Can you work these out from the model? Positions are in its coordinate system, mm. A direction names the side the tool comes from. Round coordinates to 2 decimals unless told otherwise and drop trailing zeros. Order: outer loops, then holes, each group sorted by start corner. A loop starts at its lowest first (then second) coordinate and runs counter-clockwise, first axis right, second up. Notation, with made-up numbers: M -25,9.5 L -8,9.5 A15 cw -8,27.5 Z; hole C 41,63.25 d4. An arc over 180 degrees is marked long. Answer as a JSON object with one key per item and string values. Group by question number.
```python
from build123d import *

# Parameters (mm, degrees)
SKIZZE1_R                       = 23.4
SKIZZE1_R_2                     = 1
LINEAR_AUSTRAGEN1_DEPTH         = 2.2
SKIZZE3_R                       = 1.75
SCHNITT_LINEAR_AUSTRAGEN3_DEPTH = 34.165644875
SKETCH1_R                       = 5
CUT_EXTRUDE1_DEPTH              = 3


with BuildPart() as part:
    # Skizze1 → Linear austragen1 (new body)
    with BuildSketch(Plane.XY):
        Circle(SKIZZE1_R)
        with Locations((6.643865379, 20.4477151)):
            Circle(SKIZZE1_R_2, mode=Mode.SUBTRACT)
        with Locations((17.393865379, 12.637382924)):
            Circle(SKIZZE1_R_2, mode=Mode.SUBTRACT)
        with Locations((17.393865379, -12.637382924)):
            Circle(SKIZZE1_R_2, mode=Mode.SUBTRACT)
        with Locations((-6.643865379, 20.4477151)):
            Circle(SKIZZE1_R_2, mode=Mode.SUBTRACT)
        with Locations((6.643865379, -20.4477151)):
            Circle(SKIZZE1_R_2, mode=Mode.SUBTRACT)
        with Locations((-6.643865379, -20.4477151)):
            Circle(SKIZZE1_R_2, mode=Mode.SUBTRACT)
        with Locations((-17.393865379, -12.637382924)):
            Circle(SKIZZE1_R_2, mode=Mode.SUBTRACT)
        with Locations((-17.393865379, 12.637382924)):
            Circle(SKIZZE1_R_2, mode=Mode.SUBTRACT)
        with BuildLine():
            ThreePointArc((14.720859381, 11.20474449), (0, 18.5), (-14.720859381, 11.20474449))
            ThreePointArc((-14.720859381, 11.20474449), (-14.883940446, 9.033399462), (-12.967323579, 8))
            ThreePointArc((-12.967323579, 8), (0, 8.526339105), (12.967323579, 8))
            ThreePointArc((12.967323579, 8), (14.883940446, 9.033399462), (14.720859381, 11.20474449))
        make_face(mode=Mode.SUBTRACT)
        with BuildLine():
            ThreePointArc((-14.720859381, -11.20474449), (0, -18.5), (14.720859381, -11.20474449))
            ThreePointArc((14.720859381, -11.20474449), (14.883940446, -9.033399462), (12.967323579, -8))
            ThreePointArc((12.967323579, -8), (0, -8.526339105), (-12.967323579, -8))
            ThreePointArc((-12.967323579, -8), (-14.883940446, -9.033399462), (-14.720859381, -11.20474449))
        make_face(mode=Mode.SUBTRACT)
    extrude(amount=LINEAR_AUSTRAGEN1_DEPTH)

    # Skizze3 → Schnitt-Linear austragen3 (cut, through all)
    with BuildSketch(Plane.XY.offset(2.2)):
        with Locations((12.5, 0)):
            Circle(SKIZZE3_R)
        with Locations(Location((-12.5, 0, 0), (0, 0, 180))):
            Circle(SKIZZE3_R)
        with BuildLine():
            Line((-7.295576741, 5.75), (7.295576741, 5.75))
            ThreePointArc((7.295576741, 5.75), (9.59371007, 4.678362829), (10.25, 2.229055467))
            Line((10.25, 2.229055467), (9.280201606, -3.270944533))
            ThreePointArc((9.280201606, -3.270944533), (8.254141176, -5.048133329), (6.325778347, -5.75))
            Line((6.325778347, -5.75), (-6.325778347, -5.75))
            ThreePointArc((-6.325778347, -5.75), (-8.254141176, -5.048133329), (-9.280201606, -3.270944533))
            Line((-9.280201606, -3.270944533), (-10.25, 2.229055467))
            ThreePointArc((-10.25, 2.229055467), (-9.59371007, 4.678362829), (-7.295576741, 5.75))
        make_face()
    extrude(amount=-SCHNITT_LINEAR_AUSTRAGEN3_DEPTH, mode=Mode.SUBTRACT)

    # Sketch1 → Cut-Extrude1 (cut)
    with BuildSketch(Plane.XY):
        with Locations((-25, 0)):
            Circle(SKETCH1_R)
        with Locations((25, 0)):
            Circle(SKETCH1_R)
    extrude(amount=CUT_EXTRUDE1_DEPTH, mode=Mode.SUBTRACT)


solid = part.part
```
1) For pin 1 (1.2 mm diameter, centred on x = -6.64, y = 20.45, fed in from -Z); pin 2 (1.1 mm diameter, centred on x = -1.5, z = 1.5, fed in from +Y), each with a flat end and sliding along its axis, tell me the tip position at first contact or that it passes through.
2) Which directions (+Z, -Z, +X, -X, +Y, -Y) give clear straight access to the entire face, cutting with the end or side of a thin tool? Please do faces 1 (the face through (-14.9, 9.06, 1.08)), 2 (the face through (0.45, 23.396, 1.085)).
3) If we section it at C-C on y = 0: Write out the boundary of the cut face in (x, z), plus the area to 3 significant figures.
4) If we section it at A-A on x = -2.5: Write out the boundary of the cut face in (y, z).
5) If we section it at B-B on y = -10: Write out the boundary of the cut face in (x, z), plus the area to 3 significant figures.
6) We'd pull the mould along X, two halves only. Please class faces 3 (the face through (0, 5.75, 1)), 4 (the face through (-20, 0, 1)), 5 (the face through (7.105, -21.335, 1.085)), 6 (the face through (20, 0, 1)): +X half, -X half, draft (parallel to the pull), parting line (faces both ways), or undercut.
7) If we section it at D-D on z = 1.25: Count the separate pieces of the cut face and the enclosed holes in it, plus the area to 3 significant figures.
8) I need wall thicknesses on line 1 along Y through (x, z) = (-0.5, 1.9); line 2 along Y through (x, z) = (9, 1.2); line 3 along Y through (x, z) = (6, 0.8). Which ranges of each line are inside material? Lowest first, please.
Findings:
{
 "1": {"pin 1": "passes through", "pin 2": "stops at y = 23.38"},
 "2": {"face 1": "+Z, -Z", "face 2": "+Z, -Z, +Y"},
 "3": {"outline": "M -20,0 L -14.25,0 L -14.25,2.2 L -20,2.2 Z; M -10.75,0 L -9.86,0 L -9.86,2.2 L -10.75,2.2 Z; M 9.86,0 L 10.75,0 L 10.75,2.2 L 9.86,2.2 Z; M 14.25,0 L 20,0 L 20,2.2 L 14.25,2.2 Z", "area": "29.2 mm^2"},
 "4": {"outline": "M -23.27,0 L -18.33,0 L -18.33,2.2 L -23.27,2.2 Z; M -8.51,0 L -5.75,0 L -5.75,2.2 L -8.51,2.2 Z; M 5.75,0 L 8.51,0 L 8.51,2.2 L 5.75,2.2 Z; M 18.33,0 L 23.27,0 L 23.27,2.2 L 18.33,2.2 Z"},
 "5": {"outline": "M -21.16,0 L -15.13,0 L -15.13,2.2 L -21.16,2.2 Z; M 15.13,0 L 21.16,0 L 21.16,2.2 L 15.13,2.2 Z", "area": "26.5 mm^2"},
 "6": {"face 3": "undercut", "face 4": "-X half", "face 5": "undercut", "face 6": "+X half"},
 "7": {"separate pieces": "1", "enclosed holes": "13", "area": "941 mm^2"},
 "8": {"line 1": "y = -23.39 to -18.49, -8.53 to -5.75, 5.75 to 8.53, 18.49 to 23.39", "line 2": "y = -21.6 to -16.16, -8.27 to -4.11, 5.22 to 8.27, 16.16 to 21.6", "line 3": "y = -22.62 to -21.21, -19.68 to -17.5, -8.41 to -5.75, 5.75 to 8.41, 17.5 to 19.68, 21.21 to 22.62"}
}
